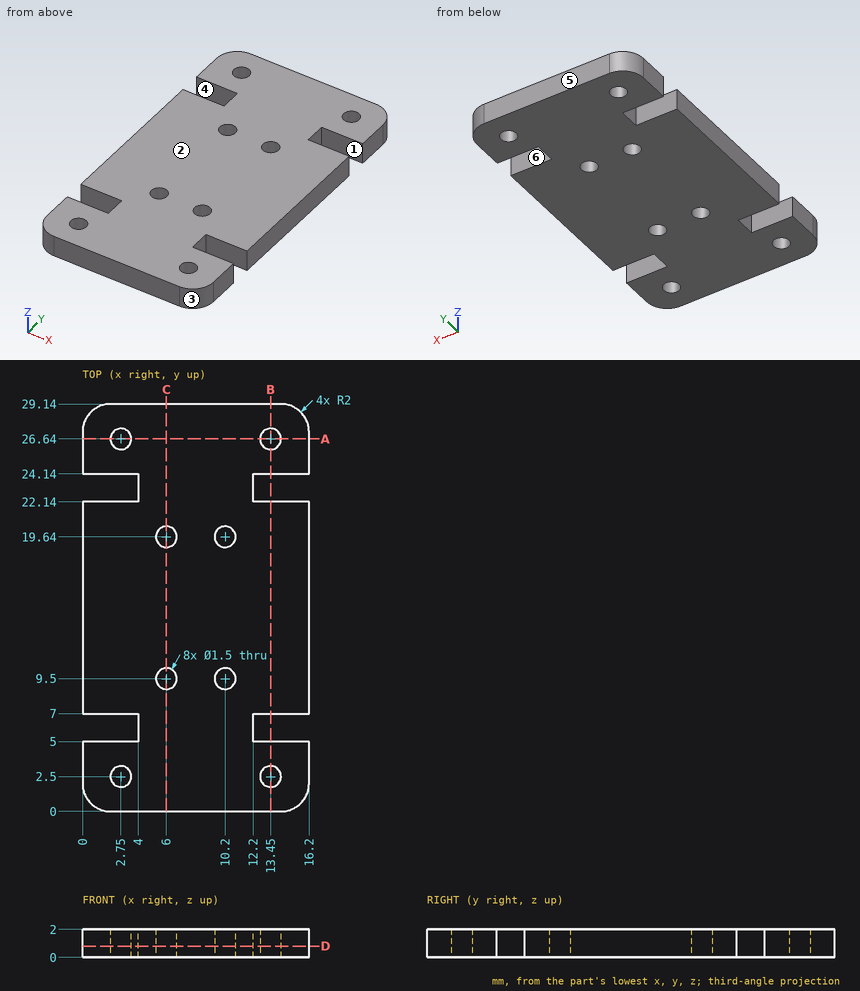
Design review of the part shown in the three views and the two pictorial views. Dimensions are in mm from the part's minimum x, y and z. A direction names the side the tool comes from. Coordinates: 2 decimals unless noted, no trailing zeros. Order: outer loops, then holes, each group sorted by start corner. A loop starts at its lowest first (then second) coordinate and runs counter-clockwise, first axis right, second up. Notation, with made-up numbers: (-12, -29) - (38, -29) arc R4 cw to (38, -22) - close; hole circle Ø11 at (9.5, 35). An arc over 180 degrees is marked (long way). One line per question, with ' | ' between items.
Q1. The part is to be moulded in two halves that separate along Y. For the marked faces 1, 2 and 3, say which applies: +Y half, -Y half, draft (parallel to the pull), parting line (faces both ways), or undercut.
Answer key:
face 1: undercut | face 2: draft | face 3: -Y half
Q2. For the marked faces 4, 5 and 6, list the 3-axis set-ups (+Z, -Z, +X, -X, +Y, -Y) from which the entire face can be reached by the end or side of a thin tool; tool diameter is ignored.
Answer key:
face 4: +Z, -Z, -X | face 5: +Z, -Z, +X, -X, +Y | face 6: +Z, -Z, +X
Q3. To check wall thickness, follow line 1 along Y through (x, z) = (6, 0.9); line 2 along Y through (x, z) = (2.75, 1.6); line 3 along Y through (x, z) = (1.5, 0.3). State the ranges of each line that lie inside material, in increasing order.
Answer key:
line 1: y = 0 to 8.75, 10.25 to 18.89, 20.39 to 29.14 | line 2: y = 0 to 1.75, 3.25 to 5, 7 to 22.14, 24.14 to 25.89, 27.39 to 29.14 | line 3: y = 0.06 to 5, 7 to 22.14, 24.14 to 29.08
Q4. Clearance check with flat-ended pins moving along their axes: pin 1 Ø0.6 at (x, z) = (15, 1) entering from +Y; pin 2 Ø0.6 at (y, z) = (6, 1) entering from -X; pin 3 Ø0.6 at (x, z) = (1.5, 1) entering from -Y. State where each tip first meets the part, or that it passes through.
Answer key:
pin 1: stops at y = 29.08 | pin 2: stops at x = 4 | pin 3: stops at y = 0.01
Q5. Consider section A-A, the plane y = 26.64. Give the boundary of the cut face in (x, z), then the cut area to 3 significant figures.
Answer key:
outline: (0, 0) - (2, 0) - (2, 2) - (0, 2) - close; (3.5, 0) - (12.7, 0) - (12.7, 2) - (3.5, 2) - close; (14.2, 0) - (16.2, 0) - (16.2, 2) - (14.2, 2) - close | area: 26.4 mm2
Q6. Consider section D-D, the plane z = 0.8. Give the number of separate pieces and of enclosed holes in the cut face, then the cut area to 3 significant figures.
Answer key:
separate pieces: 1 | enclosed holes: 8 | area: 422 mm2
Q7. Consider section B-B, the plane x = 13.45. Give the boundary of the cut face in (y, z).
Answer key:
outline: (0, 0) - (1.75, 0) - (1.75, 2) - (0, 2) - close; (3.25, 0) - (5, 0) - (5, 2) - (3.25, 2) - close; (7, 0) - (22.14, 0) - (22.14, 2) - (7, 2) - close; (24.14, 0) - (25.89, 0) - (25.89, 2) - (24.14, 2) - close; (27.39, 0) - (29.14, 0) - (29.14, 2) - (27.39, 2) - close
Q8. Consider section C-C, the plane x = 6. Give the boundary of the cut face in (y, z).
Answer key:
outline: (0, 0) - (8.75, 0) - (8.75, 2) - (0, 2) - close; (10.25, 0) - (18.89, 0) - (18.89, 2) - (10.25, 2) - close; (20.39, 0) - (29.14, 0) - (29.14, 2) - (20.39, 2) - close
